Part print with two shaded views. Sizes in mm from the minimum x, y, z corner. A direction names the side the tool comes from. Round coordinates to 2 decimals unless told otherwise and drop trailing zeros. Loops run counter-clockwise (first coordinate to the right, second up) from the corner with the lowest first, then second, coordinate; pieces in that order, holes last. Notation, with made-up numbers: (0, -34) -> (22, -34) arc R5 ccw to (22, -29) -> close; hole circle Ø11 at (-34, 4.5). An arc over 180 degrees is marked (long way). Use a Markdown table: item, result. Add a question column.
Item 1: Two-plate mould, pull along X, no slides. Class the marked faces 1, 2 and 3: pulls with the +X half, pulls with the -X half, needs draft (parallel to the pull), parting line crosses it, or undercut.
Item 2: Probe line 1 (Y direction, x = 0.4, z = 43.5); line 2 (X direction, y = 10.5, z = 25); line 3 (Z direction, x = 101.55, y = 58.5). List the from-to ranges inside material, lowest first. Write a range as [from, to].
Item 3: Cut at D-D, the plane y = 31.5. List the corners of the cut face in (x, z), plus the area to 3 significant figures.
Item 4: Cut at B-B, the plane y = 54. List the corners of the cut face in (x, z).
Item 5: Which spindle directions (+Z, -Z, +X, -X, +Y, -Y) get a long thin tool onto all of the face, cutting with end or side? Do the marked faces 4 and 5. Say none if no direction does.
Item 6: Cut at C-C, the plane z = 8. List the corners of the cut face in (x, y), plus the area to 3 significant figures.
Item 7: Cut at A-A, the plane x = 14.5. List the corners of the cut face in (y, z).
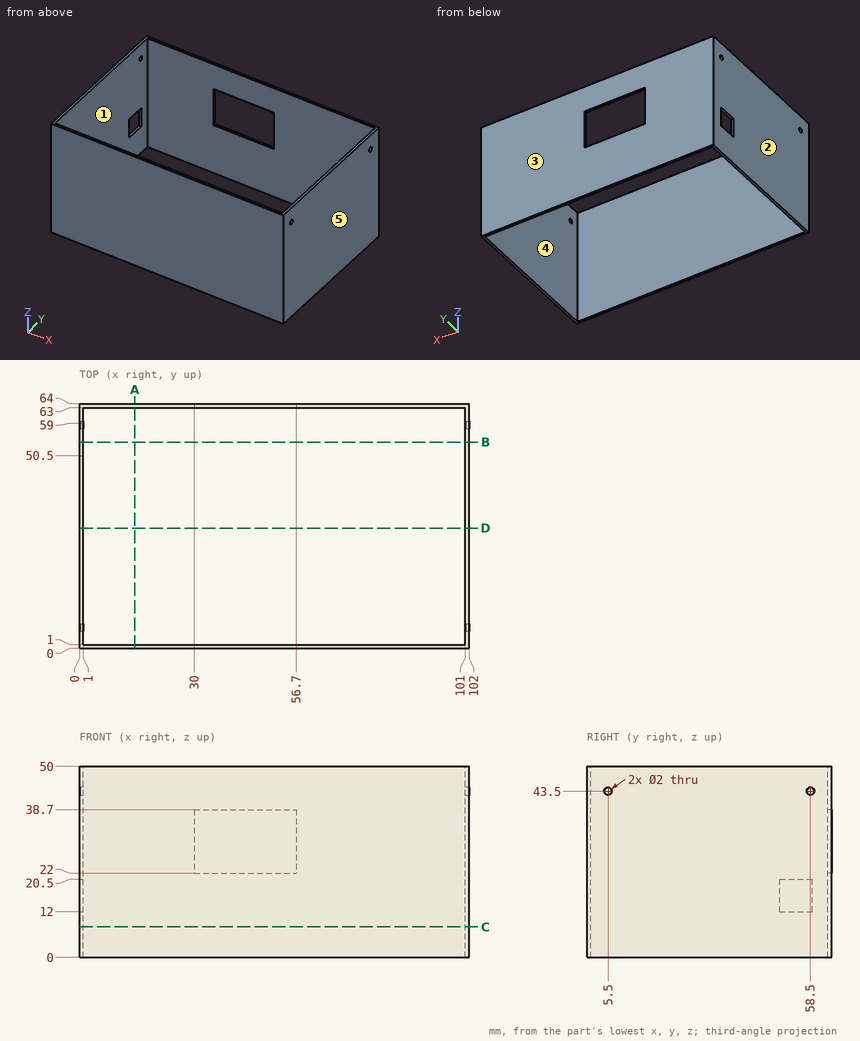
A:
| question | item | result |
|---|---|---|
| 1 | face 1 | undercut |
| 1 | face 2 | pulls with the -X half |
| 1 | face 3 | needs draft |
| 2 | line 1 | y = [0, 4.5], [6.5, 57.5], [59.5, 64] |
| 2 | line 2 | x = [0, 1], [101, 102] |
| 2 | line 3 | z = [0, 42.5], [44.5, 50] |
| 3 | outline | (0, 0) -> (1, 0) -> (1, 50) -> (0, 50) -> close; (101, 0) -> (102, 0) -> (102, 50) -> (101, 50) -> close |
| 3 | area | 100 mm^2 |
| 4 | outline | (0, 0) -> (1, 0) -> (1, 12) -> (0, 12) -> close; (0, 20.5) -> (1, 20.5) -> (1, 50) -> (0, 50) -> close; (101, 0) -> (102, 0) -> (102, 50) -> (101, 50) -> close |
| 5 | face 4 | +Z, -Z |
| 5 | face 5 | +Z, -Z, +X, +Y, -Y |
| 6 | outline | (0, 0) -> (102, 0) -> (102, 64) -> (0, 64) -> close; hole (1, 1) -> (101, 1) -> (101, 63) -> (1, 63) -> close |
| 6 | area | 328 mm^2 |
| 7 | outline | (0, 0) -> (1, 0) -> (1, 50) -> (0, 50) -> close; (63, 0) -> (64, 0) -> (64, 50) -> (63, 50) -> close |
